from build123d import *

# Parameters (mm, degrees)
REVOLVE_1_ANGLE     = 180
SKETCH_2_R          = 1.5
EXTRUDE_1_DEPTH     = 3
FILLET_1_R          = 0.4
SKETCH_3_OUTSIDE_W  = 15.25
SKETCH_3_OUTSIDE_H  = 15.25
SKETCH_3_OUTSIDE_R  = 2.5
CUT_EXTRUDE_1_DEPTH = 43
SKETCH_4_W          = 2.409556496
SKETCH_4_H          = 0.8
CUT_EXTRUDE_2_DEPTH = 21.5


with BuildPart() as part:
    # 草图1 → 旋转1 (revolve)
    with BuildSketch(Plane(origin=(0, 0, 0), x_dir=(0, 0, -1), z_dir=(1, 0, 0))):
        with BuildLine():
            Line((0, 5), (0, -5))
            ThreePointArc((0, -5), (-5, 0), (0, 5))
        make_face()
    revolve(axis=Axis((0, 5, 0), (0, -1, 0)), revolution_arc=REVOLVE_1_ANGLE)

    # 草图2 → 凸台-拉伸1 (add)
    with BuildSketch(Plane(origin=(0, 0, 0), x_dir=(0, 0, -1), z_dir=(1, 0, 0))):
        with Locations(Location((0, 0, 0), (0, 0, 180))):
            Circle(SKETCH_2_R)
    extrude(amount=EXTRUDE_1_DEPTH)

    # 圆角1
    fillet_1_edges = [part.edges().sort_by_distance(p)[0] for p in [
        (0, 0, -1.5),
        (3, 0, -1.5),
    ]]
    fillet(fillet_1_edges, radius=FILLET_1_R)

    # 草图3 outside → 切除-拉伸1 (cut)
    with BuildSketch(Plane(origin=(0, 0, 0), x_dir=(0, 0, -1), z_dir=(1, 0, 0))):
        Rectangle(SKETCH_3_OUTSIDE_W, SKETCH_3_OUTSIDE_H)
        Circle(SKETCH_3_OUTSIDE_R, mode=Mode.SUBTRACT)
    extrude(amount=-CUT_EXTRUDE_1_DEPTH, mode=Mode.SUBTRACT)

    # 草图4 → 切除-拉伸2 (cut, symmetric)
    with BuildSketch(Plane.XY):
        with Locations((-4.388752566, 0)):
            Rectangle(SKETCH_4_W, SKETCH_4_H)
    extrude(amount=CUT_EXTRUDE_2_DEPTH, both=True, mode=Mode.SUBTRACT)


solid = part.part
Check sheet for the modelled part. Datum: model origin and axes. Units: mm. A direction names the side the tool comes from. Coordinates: 2 decimals unless noted, no trailing zeros. Write each loop counter-clockwise with the first axis right and the second up, starting at its lowest first coordinate (ties: lowest second). Pieces come first, ordered by that corner, then holes.
Item 1: Depth check by flat-ended pin: pin 1 Ø1 at (y, z) = (-1, 1.5) entering from +X; pin 2 Ø2 at (x, y) = (0.5, -1.5) entering from -Z; pin 3 Ø1.5 at (y, z) = (-1.5, -1) entering from -X. Enter the tip coordinate at first touch or a pass-through.
Numbers:
pin 1: stops at x = 2.94
pin 2: stops at z = -2.42
pin 3: stops at x = -4.89
Item 2: Cross-section at A-A on y = 0. Record the boundary of the cut face in (x, z), then the cut area to 3 significant figures.
Numbers:
outline: (-3.18, -2.5) - (0, -2.5) - (0, -1.9) arc R0.4 cw to (0.4, -1.5) - (2.6, -1.5) arc R0.4 ccw to (3, -1.1) - (3, 1.1) arc R0.4 ccw to (2.6, 1.5) - (0.4, 1.5) arc R0.4 cw to (0, 1.9) - (0, 2.5) - (-3.18, 2.5) - close
area: 24.9 mm2
Item 3: Cross-section at C-C on x = -4. Record the boundary of the cut face in (y, z), then the cut area to 3 significant figures.
Numbers:
outline: (-0.4, -2.47) - (-0.4, 2.47) arc R2.5 ccw to start; (0.4, -2.47) arc R2.5 ccw to (0.4, 2.47) - close
area: 15.7 mm2
Item 4: Scan lines: probe 1 along Y at (x, z) = (-3.75, 2); probe 2 along Y at (x, z) = (-3.5, -0.1); probe 3 along X at (y, z) = (-1.3, 1.25). Record each from-to range of solid material in increasing order.
Numbers:
probe 1: y = -1.5 to -0.4, 0.4 to 1.5
probe 2: y = -2.5 to -0.4, 0.4 to 2.5
probe 3: x = -4.66 to 0.01
Item 5: Access from +Z, -Z, +X, -X, +Y, -Y to the whole of each face (thin tool, end or side, straight path). Record for faces 1 (the face through (0, 1, 2)), 2 (the face through (-3.184, 0, 0)).
Numbers:
face 1: +X
face 2: +Z, -Z, -X
Item 6: Cross-section at D-D on x = 1.25. Record the boundary of the cut face in (y, z).
Numbers:
outline: circle Ø3 at (0, 0)
Item 7: Mould release check, pull along Y, two halves, no side actions. Record for faces 3 (the face through (-4, -0.4, 0)), 4 (the face through (-2.135, 0.751, -2.385)), 5 (the face through (3, 0, 0)): released by +Y, released by -Y, zero draft, split by the parting line, or undercut.
Numbers:
face 3: undercut
face 4: split by the parting line
face 5: zero draft
Item 8: Cross-section at B-B on z = 0. Record the boundary of the cut face in (x, y), then the cut area to 3 significant figures.
Numbers:
outline: (-4.98, -0.4) arc R5 ccw to (-4.33, -2.5) - (0, -2.5) - (0, -1.9) arc R0.4 cw to (0.4, -1.5) - (2.6, -1.5) arc R0.4 ccw to (3, -1.1) - (3, 1.1) arc R0.4 ccw to (2.6, 1.5) - (0.4, 1.5) arc R0.4 cw to (0, 1.9) - (0, 2.5) - (-4.33, 2.5) arc R5 ccw to (-4.98, 0.4) - (-3.18, 0.4) - (-3.18, -0.4) - close
area: 31.5 mm2
